Could you check a few things on this model? Use its own coordinates, in mm. Round coordinates to 2 decimals unless told otherwise and drop trailing zeros. Write each loop counter-clockwise with the first axis right and the second up, starting at its lowest first coordinate (ties: lowest second). Pieces come first, ordered by that corner, then holes. Notation, with made-up numbers: (6.25, 22) -> (43.25, 22) arc R17 cw to (43.25, 55) -> close; hole circle Ø2 at (78, 67.5). An arc over 180 degrees is marked (long way). Return JSON: item names as keys, results as strings.
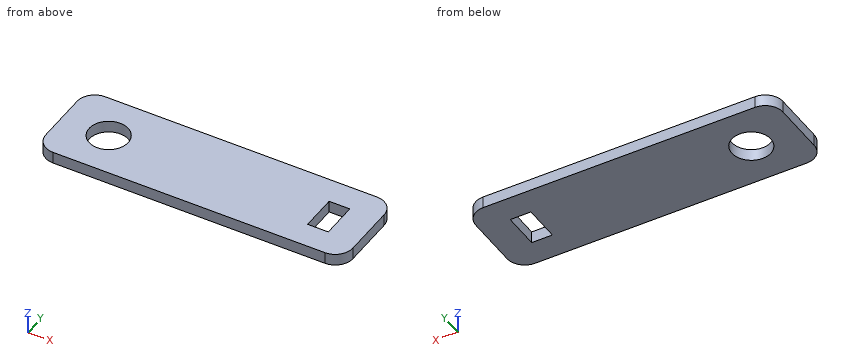
from build123d import *

# Parameters (mm, degrees)
SKETCH_W   = 52
SKETCH_H   = 15
SKETCH_R   = 3.3
SKETCH_W_2 = 3.5
SKETCH_H_2 = 6.2
PAD_DEPTH  = 2
FILLET_R   = 3


with BuildPart() as part:
    # Sketch → Pad (new body)
    with BuildSketch(Plane.XY):
        Rectangle(SKETCH_W, SKETCH_H)
        with Locations((-18, 0)):
            Circle(SKETCH_R, mode=Mode.SUBTRACT)
        with Locations((19.25, 0)):
            Rectangle(SKETCH_W_2, SKETCH_H_2, mode=Mode.SUBTRACT)
    extrude(amount=PAD_DEPTH)

    # Fillet
    fillet_edges = [part.edges().sort_by_distance(p)[0] for p in [
        (26, -7.5, 1),
        (26, 7.5, 1),
        (-26, 7.5, 1),
        (-26, -7.5, 1),
    ]]
    fillet(fillet_edges, radius=FILLET_R)


solid = part.part
1) Will this pin go through, and if not, where does the flat tip stop? pin 1 Ø1 at (y, z) = (-5.5, 1) entering from -X.
Return value:
{"pin 1": "x = -25.96"}
2) I want a section at A-A, the plane y = 0. Please give me the cut outline in (x, z), and give its area (3 significant figures).
Return value:
{"outline": "(-26, 0) -> (-21.3, 0) -> (-21.3, 2) -> (-26, 2) -> close; (-14.7, 0) -> (17.5, 0) -> (17.5, 2) -> (-14.7, 2) -> close; (21, 0) -> (26, 0) -> (26, 2) -> (21, 2) -> close", "area": "83.8 mm²"}
3) I want a section at C-C, the plane z = 0.4. Please give me the cut outline in (x, y).
Return value:
{"outline": "(-26, -4.5) arc R3 ccw to (-23, -7.5) -> (23, -7.5) arc R3 ccw to (26, -4.5) -> (26, 4.5) arc R3 ccw to (23, 7.5) -> (-23, 7.5) arc R3 ccw to (-26, 4.5) -> close; hole circle Ø6.6 at (-18, 0); hole (17.5, -3.1) -> (21, -3.1) -> (21, 3.1) -> (17.5, 3.1) -> close"}
4) I want a section at D-D, the plane x = -18. Please give me the cut outline in (y, z).
Return value:
{"outline": "(-7.5, 0) -> (-3.3, 0) -> (-3.3, 2) -> (-7.5, 2) -> close; (3.3, 0) -> (7.5, 0) -> (7.5, 2) -> (3.3, 2) -> close"}
5) I want a section at B-B, the plane x = 18. Please give me the cut outline in (y, z), and give its area (3 significant figures).
Return value:
{"outline": "(-7.5, 0) -> (-3.1, 0) -> (-3.1, 2) -> (-7.5, 2) -> close; (3.1, 0) -> (7.5, 0) -> (7.5, 2) -> (3.1, 2) -> close", "area": "17.6 mm²"}
6) If I drill on probe 1 along Y at (x, z) = (-18, 1.35); probe 2 along X at (y, z) = (2.5, 0.45); probe 3 along X at (y, z) = (3, 1), over which ranges is the centre line in solid material (lowest first)? Write a range as [from, to].
Return value:
{"probe 1": "[-7.5, -3.3], [3.3, 7.5]", "probe 2": "[-26, -20.15], [-15.85, 17.5], [21, 26]", "probe 3": "[-26, -19.37], [-16.63, 17.5], [21, 26]"}
